Can you work these out from the model? Positions are in its coordinate system, mm. Give positions to 0.01 mm unless a question says otherwise; leave off trailing zeros. Order: outer loops, then holes, each group sorted by start corner. A loop starts at its lowest first (then second) coordinate and runs counter-clockwise, first axis right, second up.
Item 1: I want a section at B-B, the plane x = -35. Write out the boundary of the cut face in (y, z), then the cut area to 3 significant figures.
Item 2: I want a section at A-A, the plane y = 22. Write out the boundary of the cut face in (x, z).
Item 3: If I drill on line 1 along Y through (x, z) = (-0.5, 1); line 2 along Y through (x, z) = (-20, 4.5); line 3 along X through (y, z) = (23, 7.75), over which ranges is the centre line in solid material (lowest first)?
Item 4: I'm going to push flat-ended pins straight in: pin 1 Ø2 at (y, z) = (31.5, 3.5) entering from +X; pin 2 Ø2 at (x, z) = (-26.5, 2) entering from +Y; pin 3 Ø5 at (x, z) = (-18, 5) entering from +Y. Where does each tip first touch, or does it pass through?
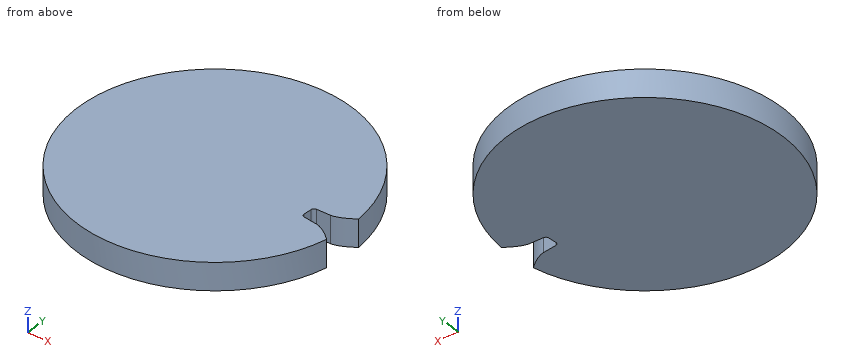
```python
from build123d import *

# Parameters (mm, degrees)
SKETCH2_R               = 50
BOSS_EXTRUDE1_DEPTH     = 10
CUT_EXTRUDE1_DEPTH      = 72.414284285
CUT_EXTRUDE1_DEPTH_BACK = 72.414284285
FILLET2_R               = 1.1


with BuildPart() as part:
    # Sketch2 → Boss-Extrude1 (new body)
    with BuildSketch(Plane.XY):
        Circle(SKETCH2_R)
    extrude(amount=BOSS_EXTRUDE1_DEPTH)

    # Sketch4 → Cut-Extrude1 (cut, two sides: drawn at the far end of the back side and taken through both)
    with BuildSketch(Plane.XY.offset(10).offset(-CUT_EXTRUDE1_DEPTH_BACK)):
        with BuildLine():
            add(Edge.make_bspline(
                [(42.286167935, 0), (42.300623625, 0.000207972), (42.341158058, 0.001435323), (42.417735849, 0.006298791), (42.542526621, 0.017843628), (42.701219946, 0.037852947), (42.905849783, 0.069790126), (43.146163964, 0.115211019), (43.409330629, 0.17327731), (43.694480037, 0.245219326), (43.977805099, 0.324724197), (44.259247021, 0.411205938), (44.538460268, 0.503808989), (44.875197444, 0.623574823), (45.276841168, 0.777725041), (45.742862789, 0.973159706), (46.267095665, 1.212747198), (46.796326187, 1.475938928), (47.312791354, 1.750494209), (47.829241884, 2.045617008), (48.325100599, 2.343712939), (48.834136207, 2.671254069), (49.264664533, 2.95849553), (49.608043611, 3.202248044), (49.805138833, 3.344334313), (49.884141613, 3.401825328)],
                knots=[0, 0, 0, 0, 0, 0.005376749, 0.015083688, 0.02853182, 0.04661014, 0.064854849, 0.092110525, 0.119476176, 0.146842496, 0.174208854, 0.201574956, 0.228941013, 0.256307345, 0.307035032, 0.361767352, 0.416499661, 0.471231937, 0.525964282, 0.580696616, 0.635428982, 0.690161387, 0.744893688, 0.782595304, 0.782595304, 0.782595304, 0.782595304, 0.782595304], degree=4))
            Line((42.286167935, 0), (36.036167935, 0))
            Line((36.036167935, 0), (35.65943594, -5.197117271))
            Line((35.65943594, -5.197117271), (41.844096723, -6.098488999))
            add(Edge.make_bspline(
                [(41.844096723, -6.098488999), (41.858371296, -6.100779588), (41.898304962, -6.107839963), (41.973380782, -6.123696596), (42.095201966, -6.153118), (42.249350534, -6.195804805), (42.447235152, -6.256919711), (42.678486444, -6.336523746), (42.930527603, -6.431936755), (43.202320541, -6.544250768), (43.471217494, -6.663785466), (43.737244794, -6.78995251), (44.000183905, -6.921855451), (44.316128172, -7.088933279), (44.691341539, -7.299396816), (45.124305757, -7.559997748), (45.608504976, -7.872685118), (46.094245403, -8.209450717), (46.565715083, -8.555620057), (47.034204041, -8.922139787), (47.481887674, -9.288631826), (47.938363873, -9.686161599), (48.322965525, -10.03249073), (48.627600964, -10.323216938), (48.802144091, -10.492242768), (48.87202963, -10.560526495)],
                knots=[0, 0, 0, 0, 0, 0.005376749, 0.015083688, 0.02853182, 0.04661014, 0.064854849, 0.092110525, 0.119476176, 0.146842496, 0.174208854, 0.201574956, 0.228941013, 0.256307345, 0.307035032, 0.361767352, 0.416499661, 0.471231937, 0.525964282, 0.580696616, 0.635428982, 0.690161387, 0.744893688, 0.782595304, 0.782595304, 0.782595304, 0.782595304, 0.782595304], degree=4))
            ThreePointArc((48.87202963, -10.560526495), (49.717207693, -5.310297473), (50, 0))
            ThreePointArc((50, 0), (49.971027009, 1.701898846), (49.884141613, 3.401825328))
        make_face()
    extrude(amount=CUT_EXTRUDE1_DEPTH + CUT_EXTRUDE1_DEPTH_BACK, mode=Mode.SUBTRACT)

    # Fillet2
    fillet2_edges = [part.edges().sort_by_distance(p)[0] for p in [
        (36.036167935, 0, 5),
        (35.65943594, -5.197117271, 5),
    ]]
    fillet(fillet2_edges, radius=FILLET2_R)


solid = part.part
```
Results list:
1. outline: (-35.71, 0) - (35.71, 0) - (35.71, 10) - (-35.71, 10) - close
1. area: 714 mm2
2. outline: (-44.9, 0) - (44.9, 0) - (44.9, 10) - (-44.9, 10) - close
3. line 1: y = -50 to 50
3. line 2: y = -45.83 to 45.83
3. line 3: x = -44.4 to 44.4
4. pin 1: stops at x = 39.62
4. pin 2: stops at y = 43.01
4. pin 3: stops at y = 47.54
